from build123d import *

# Parameters (mm, degrees)
SKETCH1_W           = 90
SKETCH1_H           = 90
BOSS_EXTRUDE1_DEPTH = 5
BOSS_EXTRUDE2_DEPTH = 2005
SKETCH3_W           = 90
SKETCH3_H           = 90
CUT_EXTRUDE3_DEPTH  = 5


with BuildPart() as part:
    # Sketch1 → Boss-Extrude1 (new body)
    with BuildSketch(Plane(origin=(0, 0, 0), x_dir=(1, 0, 0), z_dir=(0, 1, 0))):
        Rectangle(SKETCH1_W, SKETCH1_H)
    extrude(amount=BOSS_EXTRUDE1_DEPTH)

    # Sketch2 → Boss-Extrude2 (add)
    with BuildSketch(Plane.XZ):
        with BuildLine():
            Line((-7.519680062, 1.976929803), (-7.419680062, 1.976929803))
            ThreePointArc((-7.419680062, 1.976929803), (-0.074747151, 7.678171432), (7.379786606, 2.121002904))
            Line((7.379786606, 2.121002904), (7.480319938, 2.121002904))
            ThreePointArc((7.480319938, 2.121002904), (-0.074676432, 7.774848109), (-7.519680062, 1.976929803))
        make_face()
    extrude(amount=BOSS_EXTRUDE2_DEPTH)

    # Sketch3 → Cut-Extrude3 (cut)
    with BuildSketch(Plane(origin=(0, 5, 0), x_dir=(1, 0, 0), z_dir=(0, 1, 0))):
        Rectangle(SKETCH3_W, SKETCH3_H)
    extrude(amount=-CUT_EXTRUDE3_DEPTH, mode=Mode.SUBTRACT)


solid = part.part
Geometry: final body of the model. Coordinates: model frame, mm. Round coordinates to 2 decimals unless told otherwise and drop trailing zeros. Order: outer loops, then holes, each group sorted by start corner. A loop starts at its lowest first (then second) coordinate and runs counter-clockwise, first axis right, second up. Notation, with made-up numbers: (68.5, 81) -> (100.5, 81) arc R22 cw to (100.5, 110) -> close; hole circle Ø10 at (-21, -25.5). An arc over 180 degrees is marked (long way). Put each result on its own line as item: value. Start each with the question number.
Q1. Section C-C on x = 2.75. Return the cut outline in (y, z).
Q2. Section A-A on z = 3.6. Return the cut outline in (x, y), and give its area (3 significant figures).
Q3. Line query: probe 1 along X at (y, z) = (-1232.5, 6.8); probe 2 along X at (y, z) = (-1816, 6.25); probe 3 along Z at (x, y) = (6.5, -1549). Output: solid intervals per line, ascending.
Q4. First-contact query: pin 1 (1.5 mm diameter, centred on x = -0.5, z = 5, fed in from +Y); pin 2 (1 mm diameter, centred on x = 5, y = -1717.5, fed in from +Z). Flat tips, straight axial feed; report the tip coordinate or a pass-through.
Q5. Section B-B on y = -274. Return the cut outline in (x, z).
Ans:
1. outline: (-2005, 7.17) -> (0, 7.17) -> (0, 7.27) -> (-2005, 7.27) -> close
2. outline: (-6.89, -2005) -> (-6.78, -2005) -> (-6.78, 0) -> (-6.89, 0) -> close; (6.78, -2005) -> (6.89, -2005) -> (6.89, 0) -> (6.78, 0) -> close
2. area: 438 mm2
3. probe 1: x = -3.77 to -3.57, 3.57 to 3.77
3. probe 2: x = -4.63 to -4.46, 4.46 to 4.63
3. probe 3: z = 4.09 to 4.27
4. pin 1: passes through
4. pin 2: stops at z = 6.34
5. outline: (-7.52, 1.98) -> (-7.42, 1.98) arc R7.68 cw to (7.38, 2.12) -> (7.48, 2.12) arc R7.78 ccw to start
